```python
from build123d import *

# Parameters (mm, degrees)
F1_R     = 13.9916710172
F2_DEPTH = 25.4
F4_W     = 36.2210944295
F4_H     = 17.3936840147
F5_DEPTH = 36.2169072032
F6_DEPTH = 11.5376953036


with BuildPart() as f2:
    # F1 (on face) → F2 (new body)
    with BuildSketch(Plane.XY):
        Circle(F1_R)
    extrude(amount=F2_DEPTH)

    # F4 (on face) → F5 (join)
    with BuildSketch(Plane(origin=(0, -17.5722502172, 0), x_dir=(-1, 0, 0), z_dir=(0, 1, 0))):
        with Locations((0, 8.6968420073)):
            Rectangle(F4_W, F4_H)
    extrude(amount=F5_DEPTH)

    # F6 (cut): a face of the model
    f6_faces = [f2.faces().sort_by_distance(p)[0] for p in [
        (0, 0, 25.4),
    ]]
    extrude(f6_faces, amount=-F6_DEPTH, mode=Mode.SUBTRACT)


solid = f2.part
```
Geometry check sheet. Reference: the model listing, model coordinates, mm. A direction names the side the tool comes from. Round coordinates to 2 decimals unless told otherwise and drop trailing zeros. Loops run counter-clockwise (first coordinate to the right, second up) from the corner with the lowest first, then second, coordinate; pieces in that order, holes last. Notation, with made-up numbers: (20, -31.5) - (61, -31.5) arc R7 ccw to (61, -19.5) - close; hole circle Ø4 at (9, 77.5). An arc over 180 degrees is marked (long way). Write each question's results on one line, items separated by ' | '. Start each with the question number.
Q1. Gauge pin test, flat end, axial feed: P1, Ø14, axis at x = 4, y = -5.5, coming from the +Z side. Record the tip position at first contact, or that the pin passes through.
Q2. Cross-section at B-B on x = 0. Enter the section's corners in (y, z), and give its area (3 significant figures).
Q3. Cross-section at A-A on y = 0. Enter the section's corners in (x, z).
Q4. Access from +Z, -Z, +X, -X, +Y, -Y to the whole of each face (thin tool, end or side, straight path). Record for faces 1 (the flat face through (0, 0, 0)), 2 (the cylindrical face through (-1.821, 13.873, 15.653)).
Q5. Thickness scan on line 1 (Y direction, x = 0, z = 15.5); line 2 (X direction, y = 0, z = 15.95); line 3 (Y direction, x = 7.5, z = 14.5). Record the ranges inside material, lowest first. Write a range as [from, to].
Q6. Release check for a two-part mould opening along Y. For faces 3 (the flat face through (-18.111, 0, 9)), 4 (the flat face through (0, 0, 13.862)), 5 (the flat face through (0, 18.645, 9)) record: +Y half, -Y half, draft (parallel to the pull), parting line (faces both ways), or undercut.
Answers below:
1) P1: stops at z = 13.86
2) outline: (-17.57, 0) - (18.64, 0) - (18.64, 17.39) - (13.99, 17.39) - (13.99, 13.86) - (-13.99, 13.86) - (-13.99, 17.39) - (-17.57, 17.39) - close | area: 531 mm²
3) outline: (-18.11, 0) - (18.11, 0) - (18.11, 17.39) - (13.99, 17.39) - (13.99, 13.86) - (-13.99, 13.86) - (-13.99, 17.39) - (-18.11, 17.39) - close
4) face 1: -Z, +X, -X, +Y, -Y | face 2: +Z
5) line 1: y = [-17.57, -13.99], [13.99, 18.64] | line 2: x = [-18.11, -13.99], [13.99, 18.11] | line 3: y = [-17.57, -11.81], [11.81, 18.64]
6) face 3: draft | face 4: undercut | face 5: +Y half
